Verification items for the finished model (mm, model axes). A direction names the side the tool comes from. Round coordinates to 2 decimals unless told otherwise and drop trailing zeros. Order: outer loops, then holes, each group sorted by start corner. A loop starts at its lowest first (then second) coordinate and runs counter-clockwise, first axis right, second up. Notation, with made-up numbers: (-12.5, 8) -> (15.5, 8) arc R27 cw to (15.5, 42) -> close; hole circle Ø10 at (57.25, 39). An arc over 180 degrees is marked (long way). Return JSON: item names as keys, results as strings. Group by question number.
1) Scan lines: L1, parallel to Y at x = -17.75, z = 0.85; L2, parallel to Y at x = -25.5, z = 1.2; L3, parallel to X at y = -1, z = 0.55. Record each from-to range of solid material in increasing order.
2) Section check B-B on x = 17.75. Enter the section's corners in (y, z), plus the area to 3 significant figures.
3) Draft check along X on faces 1 (the cylindrical face through (16.5, -19.9, 1.5)), 2 (the flat face through (-46.75, 19, 1)), 3 (the flat face through (1, -25, 1)). Enter one of: pulls with the +X half, pulls with the -X half, needs draft (parallel to the pull), parting line crosses it, or undercut.
4) Depth check by flat-ended pin: pin 1 (3 mm diameter, centred on x = 17.75, y = -18.9, fed in from -Z); pin 2 (0.9 mm diameter, centred on x = -25, z = 1.5, fed in from +Y); pin 3 (0.9 mm diameter, centred on y = -3, z = 2, fed in from -X). Enter the tip coordinate at first touch or a pass-through.
5) Section check C-C on y = -18.9. Enter the section's corners in (x, z).
6) Section check D-D on x = -22. Enter the section's corners in (y, z).
7) Section check A-A on z = 2.55. Enter the section's corners in (x, y).
8) Tool access check on faces 4 (the flat face through (-10, 26, 2)), 5 (the flat face through (43.75, 0, 1)), 6 (the flat face through (10, 26, 2)), 7 (the flat face through (-45, 12.5, 1)). Record the directions out of +Z, -Z, +X, -X, +Y, -Y that give a thin tool (end or side, any length) a straight path to the whole face; none if there is none.
```python
from build123d import *

# Parameters (mm, degrees)
BOSS_EXTRU_1_DEPTH = 3
ESQUISSE2_W        = 20
ESQUISSE2_H        = 3
BOSS_EXTRU_2_DEPTH = 3
SKETCH1_R          = 1.6
CUT_EXTRUDE1_DEPTH = 55.576208186
SKETCH2_R          = 1.6
CUT_EXTRUDE2_DEPTH = 55.576208186
SKETCH3_R          = 1.6
CUT_EXTRUDE3_DEPTH = 55.576208186


with BuildPart() as part:
    # Esquisse1 → Boss.-Extru.1 (new body)
    with BuildSketch(Plane.XY):
        Polygon((46.75, -25), (-46.75, -25), (-46.75, -12.7), (-43.75, -12.7), (-43.75, 12.5), (-46.75, 12.5), (-46.75, 25), (-26.2, 25), (-23, 25), (23, 25), (26.2, 25), (46.75, 25), (46.75, 12.5), (43.75, 12.5), (43.75, -12.7), (46.75, -12.7), align=None)
    extrude(amount=BOSS_EXTRU_1_DEPTH)

    # Esquisse2 → Boss.-Extru.2 (add)
    with BuildSketch(Plane.XY.offset(3)):
        with Locations((0, 26.5)):
            Rectangle(ESQUISSE2_W, ESQUISSE2_H)
    extrude(amount=-BOSS_EXTRU_2_DEPTH)

    # Sketch1 → Cut-Extrude1 (cut, through all)
    with BuildSketch(Plane.XY.offset(3)):
        with Locations((-17.75, 21)):
            Circle(SKETCH1_R)
    extrude(amount=-CUT_EXTRUDE1_DEPTH, mode=Mode.SUBTRACT)

    # Sketch2 → Cut-Extrude2 (cut, through all)
    with BuildSketch(Plane(origin=(0, 0, 0), x_dir=(-1, 0, 0), z_dir=(0, 0, -1))):
        with Locations((-17.75, 21)):
            Circle(SKETCH2_R)
    extrude(amount=-CUT_EXTRUDE2_DEPTH, mode=Mode.SUBTRACT)

    # Sketch3 → Cut-Extrude3 (cut, through all)
    with BuildSketch(Plane.XY.offset(3)):
        with Locations((17.75, -18.9)):
            Circle(SKETCH3_R)
        with Locations((-17.75, -18.9)):
            Circle(SKETCH3_R)
    extrude(amount=-CUT_EXTRUDE3_DEPTH, mode=Mode.SUBTRACT)


solid = part.part
```
Check result:
{
 "1": {"L1": "-25 to -20.5, -17.3 to 19.4, 22.6 to 25", "L2": "-25 to 25", "L3": "-43.75 to 43.75"},
 "2": {"outline": "(-25, 0) -> (-20.5, 0) -> (-20.5, 3) -> (-25, 3) -> close; (-17.3, 0) -> (19.4, 0) -> (19.4, 3) -> (-17.3, 3) -> close; (22.6, 0) -> (25, 0) -> (25, 3) -> (22.6, 3) -> close", "area": "131 mm^2"},
 "3": {"face 1": "undercut", "face 2": "pulls with the -X half", "face 3": "needs draft"},
 "4": {"pin 1": "through", "pin 2": "y = 25", "pin 3": "x = -43.75"},
 "5": {"outline": "(-46.75, 0) -> (-19.35, 0) -> (-19.35, 3) -> (-46.75, 3) -> close; (-16.15, 0) -> (16.15, 0) -> (16.15, 3) -> (-16.15, 3) -> close; (19.35, 0) -> (46.75, 0) -> (46.75, 3) -> (19.35, 3) -> close"},
 "6": {"outline": "(-25, 0) -> (25, 0) -> (25, 3) -> (-25, 3) -> close"},
 "7": {"outline": "(-46.75, -25) -> (46.75, -25) -> (46.75, -12.7) -> (43.75, -12.7) -> (43.75, 12.5) -> (46.75, 12.5) -> (46.75, 25) -> (10, 25) -> (10, 28) -> (-10, 28) -> (-10, 25) -> (-46.75, 25) -> (-46.75, 12.5) -> (-43.75, 12.5) -> (-43.75, -12.7) -> (-46.75, -12.7) -> close; hole circle Ø3.2 at (-17.75, -18.9); hole circle Ø3.2 at (-17.75, 21); hole circle Ø3.2 at (17.75, -18.9); hole circle Ø3.2 at (17.75, 21)"},
 "8": {"face 4": "+Z, -Z, -X, +Y", "face 5": "+Z, -Z, +X", "face 6": "+Z, -Z, +X, +Y", "face 7": "+Z, -Z, -X"}
}
